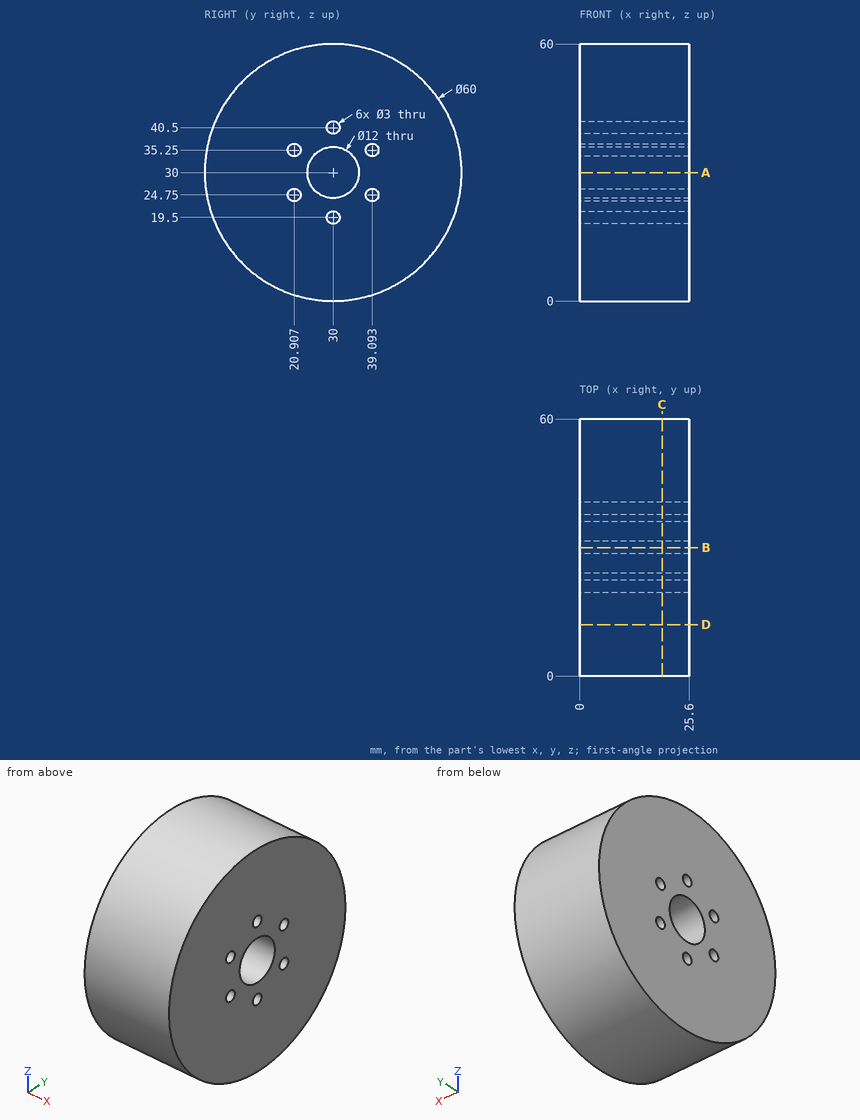
Print and shaded views of the part. All mm, measured from the part's lowest x, y and z. Coordinates: 2 decimals unless noted, no trailing zeros. Order: outer loops, then holes, each group sorted by start corner. A loop starts at its lowest first (then second) coordinate and runs counter-clockwise, first axis right, second up. Notation, with made-up numbers: M -10,16 L 14,16 A24 ccw 14,33 Z; hole C 35.5,-17.5 d10. An arc over 180 degrees is marked long. Answer as CSV lines item,"result".
1) Cut at C-C (x = 19.25). List the corners of the cut face in (y, z), then the cut area to 3 significant figures.
Verdict:
outline,"C 30,30 d60; hole C 20.91,24.75 d3; hole C 20.91,35.25 d3; hole C 30,30 d12; hole C 30,19.5 d3; hole C 30,40.5 d3; hole C 39.09,24.75 d3; hole C 39.09,35.25 d3"
area,"2,670 mm2"
2) Cut at A-A (z = 30). List the corners of the cut face in (x, y), then the cut area to 3 significant figures.
Verdict:
outline,"M 0,0 L 25.6,0 L 25.6,24 L 0,24 Z; M 0,36 L 25.6,36 L 25.6,60 L 0,60 Z"
area,"1,230 mm2"
3) Flat gauge pins, fed straight in: P1, Ø1.8, axis at y = 30, z = 19.5, coming from the +X side; P2, Ø5, axis at x = 22, y = 47.5, coming from the -Z side; P3, Ø12, axis at x = 22, y = 23, coming from the +Z side; P4, Ø8, axis at x = 19, z = 10, coming from the -Y side. Where does each tip first touch, or does it go through?
Verdict:
P1,"through"
P2,"z = 4.02"
P3,"z = 59.98"
P4,"y = 4.62"
4) Cut at B-B (y = 30). List the corners of the cut face in (x, z).
Verdict:
outline,"M 0,0 L 25.6,0 L 25.6,18 L 0,18 Z; M 0,21 L 25.6,21 L 25.6,24 L 0,24 Z; M 0,36 L 25.6,36 L 25.6,39 L 0,39 Z; M 0,42 L 25.6,42 L 25.6,60 L 0,60 Z"
5) Drill centre lines: L1, parallel to Z at x = 11.75, y = 22 (1 decimal); L2, parallel to Z at x = 8.5, y = 31 (1 decimal); L3, parallel to Y at x = 16.5, z = 30. Where is each one in solid material? Low to high. Write a range as from..to.
Verdict:
L1,"1.1..23.7, 25.8..34.2, 36.3..58.9"
L2,"0..18.4, 20.6..24.1, 35.9..39.4, 41.6..60"
L3,"0..24, 36..60"
6) Cut at D-D (y = 12). List the corners of the cut face in (x, z), then the cut area to 3 significant figures.
Verdict:
outline,"M 0,6 L 25.6,6 L 25.6,54 L 0,54 Z"
area,"1,230 mm2"
